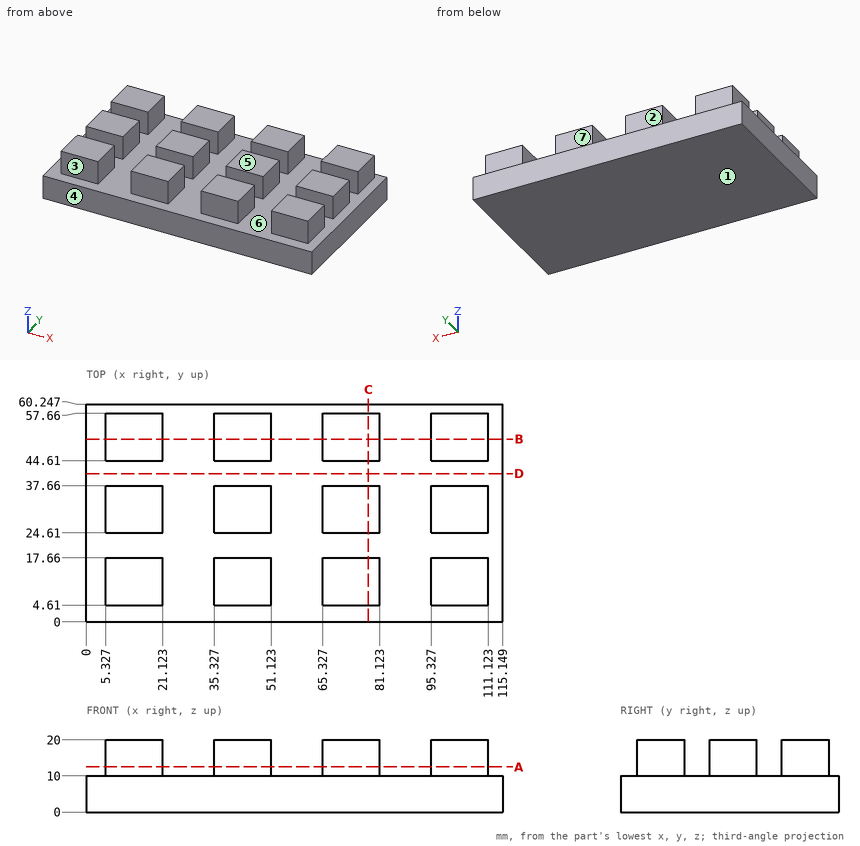
Print and shaded views of the part. All mm, measured from the part's lowest x, y and z. A direction names the side the tool comes from. Coordinates: 2 decimals unless noted, no trailing zeros. Order: outer loops, then holes, each group sorted by start corner. A loop starts at its lowest first (then second) coordinate and runs counter-clockwise, first axis right, second up. Notation, with made-up numbers: M -0.75,-15.75 L 35.25,-15.75 A12 ccw 35.25,5.25 Z; hole C -36.75,47 d8. An arc over 180 degrees is marked long. Write each question's results on one line, items separated by ' | '. Start each with the question number.
Q1. Which spindle directions (+Z, -Z, +X, -X, +Y, -Y) get a long thin tool onto all of the face, cutting with end or side? Do the marked faces 1, 2 and 3. Say none if no direction does.
Q2. Cut at C-C (x = 78). List the corners of the cut face in (y, z), then the cut area to 3 significant figures.
Q3. Cut at D-D (y = 41). List the corners of the cut face in (x, z).
Q4. Flat gauge pins, fed straight in: P1, Ø11, axis at x = 76.5, z = 14, coming from the -Y side; P2, Ø5, axis at y = 10.5, z = 17.5, coming from the +X side; P3, Ø3, axis at y = 49.5, z = 17, coming from the -X side; P4, Ø11, axis at x = 44.5, z = 16, coming from the +Y side. Where does each tip first touch, or does it go through?
Q5. Drill centre lines: probe 1 along Y at (x, z) = (7, 18); probe 2 along X at (y, z) = (56, 15); probe 3 along Z at (x, y) = (6, 19.5). Where is each one in solid material? Low to high. Write a range as from..to.
Q6. Pull direction Y, two halves, no side cores. Call the marked faces 4, 5, 6 and 7: +Y half, -Y half, draft (parallel to the pull), parting line (faces both ways), or undercut.
Q7. Cut at A-A (z = 12.5). Count the separate pieces of the cut face and the enclosed holes in it, then the cut area to 3 significant figures.
Q8. Cut at B-B (y = 50.5). List the corners of the cut face in (x, z).
Found:
1) face 1: -Z, +X, -X, +Y, -Y | face 2: +Z, +X, -X, +Y | face 3: +Z, +X, -X, -Y
2) outline: M 0,0 L 60.25,0 L 60.25,10 L 57.66,10 L 57.66,20 L 44.61,20 L 44.61,10 L 37.66,10 L 37.66,20 L 24.61,20 L 24.61,10 L 17.66,10 L 17.66,20 L 4.61,20 L 4.61,10 L 0,10 Z | area: 994 mm²
3) outline: M 0,0 L 115.15,0 L 115.15,10 L 0,10 Z
4) P1: y = 0 | P2: x = 111.12 | P3: x = 5.33 | P4: y = 57.66
5) probe 1: 4.61..17.66, 24.61..37.66, 44.61..57.66 | probe 2: 5.33..21.12, 35.33..51.12, 65.33..81.12, 95.33..111.12 | probe 3: 0..10
6) face 4: -Y half | face 5: draft | face 6: undercut | face 7: +Y half
7) separate pieces: 12 | enclosed holes: 0 | area: 2,470 mm²
8) outline: M 0,0 L 115.15,0 L 115.15,10 L 111.12,10 L 111.12,20 L 95.33,20 L 95.33,10 L 81.12,10 L 81.12,20 L 65.33,20 L 65.33,10 L 51.12,10 L 51.12,20 L 35.33,20 L 35.33,10 L 21.12,10 L 21.12,20 L 5.33,20 L 5.33,10 L 0,10 Z
